Verification items for the finished model (mm, model axes). Face numbers are marked on the shaded views. A direction names the side the tool comes from. Round coordinates to 2 decimals unless told otherwise and drop trailing zeros. Write each loop counter-clockwise with the first axis right and the second up, starting at its lowest first coordinate (ties: lowest second). Pieces come first, ordered by that corner, then holes.
Autodesk Inventor part; units mm, degrees
ref_plane "YZ Plane" through (0, 0, 0) normal (1, 0, 0) x (0, 1, 0)
ref_plane "XZ Plane" through (0, 0, 0) normal (0, 1, 0) x (-1, 0, 0)
ref_plane "XY Plane" through (0, 0, 0) normal (0, 0, 1) x (1, 0, 0)
sketch "Sketch1" plane through (0, 0, 0) normal (0, 1, 0) x (-1, 0, 0)
  line L0 (55.925, 58.5) -> (-55.925, 58.5)
  line L1 (-55.925, 58.5) -> (-55.925, -58.5)
  line L2 (-55.925, -58.5) -> (55.925, -58.5)
  line L3 (55.925, -58.5) -> (55.925, 58.5)
  line L4 (55.925, 58.5) -> (-55.925, -58.5) construction
  line L5 (-55.925, 58.5) -> (55.925, -58.5) construction
  point P0 (0, 0)
  dimension "d0" = 111.85
  dimension "d1" = 117
extrude "Extrusion1" add sketch "Sketch1" along normal blind 34.19
fillet "Fillet1" radius 2 4 edges at (0, 34.19, 58.5) (55.925, 34.19, 0) (0, 34.19, -58.5) (-55.925, 34.19, 0)
sketch "Sketch2" plane through (0, 0, 0) normal (0, -1, 0) x (1, 0, 0)
  circle A0 centre (45.425, 48) radius 5.375
  line L0 (55.925, 58.5) -> (55.925, -58.5)
  line L1 (-55.925, 58.5) -> (55.925, 58.5)
  circle A1 centre (-45.575, 48) radius 5.375
  circle A2 centre (45.425, -47) radius 5.375
  circle A3 centre (-45.575, -47) radius 5.375
  point P0 (0, 0)
  dimension "d5" = 10.75
  dimension "d6" = 10.5
  dimension "d7" = 10.5
  dimension "d10" = 91
  dimension "d13" = 95
extrude "Extrusion2" add sketch "Sketch2" along normal blind 1.5
sketch "Sketch4" plane through (0, 0, 0) normal (0, -1, 0) x (1, 0, 0)
  line L0 (-55.925, -58.5) -> (-55.925, 58.5)
  line L1 (-55.925, 58.5) -> (55.925, 58.5)
  point P0 (0, 0)
  point P1 (-42.625, 0)
  dimension "d32" = 13.3
  dimension "d33" = 58.5
hole "Hole2" at (-42.625, 0, 0) direction (0, 1, 0) diameter 3 depth 1 tip angle 118
pattern_linear "Rectangular Pattern1" count 2 spacing 84.5 along (1, 0, 0) of "Hole2"
sketch "Sketch5" plane through (55.925, 0, 58.5) normal (1, 0, 0) x (0, 0, -1)
  line L0 (34.3, 14.5) -> (47.9, 14.5)
  line L1 (47.9, 14.5) -> (47.9, 8.6)
  line L2 (47.9, 8.6) -> (34.3, 8.6)
  line L3 (34.3, 8.6) -> (34.3, 14.5)
  line L4 (34.3, 14.5) -> (47.9, 8.6) construction
  line L5 (47.9, 14.5) -> (34.3, 8.6) construction
  line L6 (52.76, 14.5) -> (66.36, 14.5)
  line L7 (66.36, 14.5) -> (66.36, 8.6)
  line L8 (66.36, 8.6) -> (52.76, 8.6)
  line L9 (52.76, 8.6) -> (52.76, 14.5)
  line L10 (52.76, 14.5) -> (66.36, 8.6) construction
  line L11 (66.36, 14.5) -> (52.76, 8.6) construction
  line L12 (0, 0) -> (117, 0)
  line L13 (0, 0) -> (0, 32.19)
  point P0 (58.5, 0)
  point P1 (41.1, 11.55)
  point P2 (59.56, 11.55)
  dimension "d37" = 13.6
  dimension "d38" = 5.9
  dimension "d39" = 13.6
  dimension "d40" = 5.9
  dimension "d41" = 8.6
  dimension "d42" = 34.3
  dimension "d43" = 4.86
  dimension "d44" = 8.6
extrude "Extrusion3" cut sketch "Sketch5" against normal blind 1.5
sketch "Sketch6" plane through (55.925, 0, 58.5) normal (1, 0, 0) x (0, 0, -1)
  line L0 (66.36, 14.5) -> (66.36, 8.6)
  line L1 (0, 0) -> (117, 0)
  point P0 (58.5, 0)
  point P1 (75.26, 12)
  dimension "d54" = 8.9
  dimension "d55" = 12
hole "Hole3" at (55.925, 12, -16.76) direction (-1, 0, 0) diameter 4.24 depth 10.688 tip angle 118
sketch "Sketch7" plane through (-55.925, 0, -58.5) normal (-1, 0, 0) x (0, 0, 1)
  line L0 (0, 0) -> (117, 0)
  line L1 (0, 0) -> (0, 32.19)
  point P0 (58.5, 0)
  point P1 (20, 9.25)
  dimension "d56" = 9.25
  dimension "d64" = 20
hole "Hole4" at (-55.925, 9.25, -38.5) direction (1, 0, 0) diameter 6.88 depth 10.688 tip angle 118
sketch "Sketch8" plane through (-55.925, 0, -58.5) normal (-1, 0, 0) x (0, 0, 1)
  line L0 (33.6837, 13.1926) -> (42.498, 13.1926)
  line L1 (46.62, 11.6426) -> (46.62, 8.31)
  line L2 (46.62, 8.31) -> (30.5, 8.31)
  line L3 (30.5, 8.31) -> (30.5, 11.6426)
  line L4 (30.5, 14.87) -> (46.62, 8.31) construction
  line L5 (46.62, 14.87) -> (30.5, 8.31) construction
  circle A0 centre (20, 9.25) radius 3.44
  line L6 (0, 0) -> (117, 0)
  line L7 (30.5, 11.6426) -> (33.6837, 13.1926)
  line L8 (42.498, 13.1926) -> (46.62, 11.6426)
  point P0 (58.5, 0)
  point P1 (38.56, 11.59)
  dimension "d65" = 16.12
  dimension "d66" = 6.56
  dimension "d67" = 10.5
  dimension "d68" = 8.31
  dimension "d69" = 1.55
  dimension "d70" = 1.55
  dimension "d71" = 8.8143
extrude "Extrusion4" cut sketch "Sketch8" against normal blind 1.5 contours L0 L8 L1 L2 L3 L7
sketch "Sketch10" plane through (-55.925, 0, -58.5) normal (-1, 0, 0) x (0, 0, 1)
  line L0 (51.62, 18.8) -> (67.17, 18.8)
  line L1 (67.17, 18.8) -> (67.17, 7.1)
  line L2 (67.17, 7.1) -> (51.62, 7.1)
  line L3 (51.62, 7.1) -> (51.62, 18.8)
  line L4 (51.62, 18.8) -> (67.17, 7.1) construction
  line L5 (67.17, 18.8) -> (51.62, 7.1) construction
  line L6 (46.62, 11.6426) -> (46.62, 8.31)
  line L7 (0, 0) -> (117, 0)
  point P0 (58.5, 0)
  point P1 (59.395, 12.95)
  dimension "d81" = 15.55
  dimension "d82" = 11.7
  dimension "d84" = 5
  dimension "d85" = 7.1
extrude "Extrusion5" cut sketch "Sketch10" against normal blind 1.5
sketch "Sketch11" plane through (-55.925, 0, -58.5) normal (-1, 0, 0) x (0, 0, 1)
  line L0 (71.57, 20.05) -> (85.87, 20.05)
  line L1 (85.87, 20.05) -> (85.87, 13.45)
  line L2 (85.87, 13.45) -> (71.57, 13.45)
  line L3 (71.57, 13.45) -> (71.57, 20.05)
  line L4 (71.57, 20.05) -> (85.87, 13.45) construction
  line L5 (85.87, 20.05) -> (71.57, 13.45) construction
  line L6 (0, 32.19) -> (117, 32.19)
  line L7 (67.17, 18.8) -> (67.17, 7.1)
  line L8 (71.57, 11.05) -> (85.87, 11.05)
  line L9 (85.87, 11.05) -> (85.87, 4.45)
  line L10 (85.87, 4.45) -> (71.57, 4.45)
  line L11 (71.57, 4.45) -> (71.57, 11.05)
  point P0 (58.5, 0)
  point P1 (78.72, 16.75)
  point P2 (79.72, 17.75)
  dimension "d88" = 14.3
  dimension "d89" = 6.6
  dimension "d90" = 12.14
  dimension "d91" = 4.4
  dimension "d92" = 14.3
  dimension "d93" = 6.6
  dimension "d94" = 2.4
  dimension "d95" = 4.4
extrude "Extrusion6" cut sketch "Sketch11" against normal blind 1.5
sketch "Sketch12" plane through (-55.925, 0, -58.5) normal (-1, 0, 0) x (0, 0, 1)
  line L0 (93.15, 19.5997) -> (99.7593, 19.5997) construction
  line L1 (93.15, 17.8293) -> (99.7593, 17.8293)
  line L2 (99.7593, 21.37) -> (93.15, 21.37)
  arc A0 (93.15, 21.37) -> (93.15, 17.8293) centre (93.15, 19.5997) ccw
  arc A1 (99.7593, 17.8293) -> (99.7593, 21.37) centre (99.7593, 19.5997) ccw
  line L3 (0, 32.19) -> (117, 32.19)
  line L4 (85.87, 20.05) -> (85.87, 13.45)
  point P0 (58.5, 0)
  point P1 (96.4547, 19.5997)
  dimension "d98" = 10.15
  dimension "d99" = 10.82
  dimension "d100" = 7.28
extrude "Extrusion7" cut sketch "Sketch12" against normal blind 1.5
sketch "Sketch13" plane through (55.925, 0, 58.5) normal (1, 0, 0) x (0, 0, -1)
  line L0 (89.56, 16.8) -> (98.76, 16.8)
  line L1 (98.76, 16.8) -> (98.76, 7.6)
  line L2 (98.76, 7.6) -> (89.56, 7.6)
  line L3 (89.56, 7.6) -> (89.56, 16.8)
  line L4 (89.56, 16.8) -> (98.76, 7.6) construction
  line L5 (98.76, 16.8) -> (89.56, 7.6) construction
  circle A0 centre (75.26, 12) radius 2.12
  line L6 (0, 0) -> (117, 0)
  point P0 (58.5, 0)
  point P1 (94.16, 12.2)
  dimension "d103" = 14.3
  dimension "d104" = 7.6
  dimension "d105" = 9.2
  dimension "d106" = 9.2
extrude "Extrusion8" add sketch "Sketch13" along normal blind 1.5 contours L0 L1 L2 L3
sketch "Sketch14" plane through (-55.925, 0, 58.5) normal (0, 0, 1) x (1, 0, 0)
  line L0 (66.65, 18.82) -> (90.15, 18.82)
  line L1 (90.15, 18.82) -> (90.15, 12.25)
  line L2 (90.15, 12.25) -> (66.65, 12.25)
  line L3 (66.65, 12.25) -> (66.65, 18.82)
  line L4 (66.65, 18.82) -> (90.15, 12.25) construction
  line L5 (90.15, 18.82) -> (66.65, 12.25) construction
  line L6 (0, 0) -> (111.85, 0)
  line L7 (111.85, 0) -> (111.85, 32.19)
  point P0 (55.925, 0)
  point P1 (78.4, 15.535)
  dimension "d109" = 23.5
  dimension "d110" = 6.57
  dimension "d111" = 12.25
  dimension "d112" = 21.7
extrude "Extrusion9" cut sketch "Sketch14" against normal blind 1.5
properties part number "NUC_model"
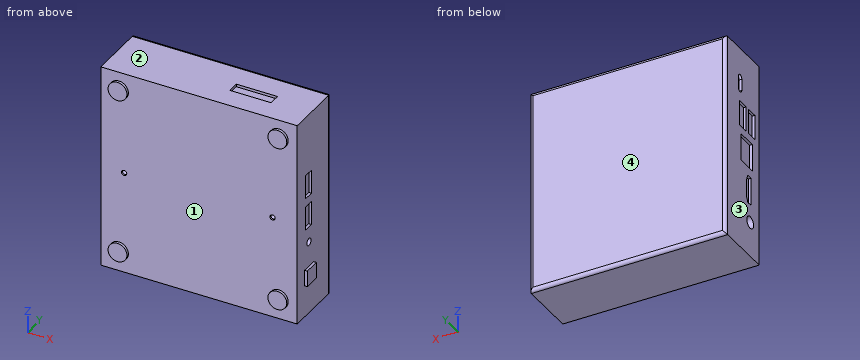
Q1. Sectioned sample at B-B (x = 28.5). Enter the section's corners in (y, z).
Recorded:
outline: (0, -58.5) - (32.19, -58.5) arc R2 ccw to (34.19, -56.5) - (34.19, 56.5) arc R2 ccw to (32.19, 58.5) - (18.82, 58.5) - (18.82, 57) - (12.25, 57) - (12.25, 58.5) - (0, 58.5) - close
Q2. Depth check by flat-ended pin: P1, Ø12, axis at x = -42, z = 9.5, coming from the -Y side; P2, Ø1.2, axis at x = -55, z = 21.5, coming from the +Y side; P3, Ø10, axis at y = 23, z = -25, coming from the +X side (3 decimals). Enter the tip coordinate at first touch or a pass-through.
Recorded:
P1: stops at y = 0
P2: stops at y = 34.13
P3: stops at x = 55.925
Q3. Sectioned sample at C-C (x = 49). Enter the section's corners in (y, z).
Recorded:
outline: (-1.5, -51.01) - (0, -51.01) - (0, -58.5) - (32.19, -58.5) arc R2 ccw to (34.19, -56.5) - (34.19, 56.5) arc R2 ccw to (32.19, 58.5) - (0, 58.5) - (0, 52.01) - (-1.5, 52.01) - (-1.5, 43.99) - (0, 43.99) - (0, -42.99) - (-1.5, -42.99) - close; hole circle Ø4.24 at (12, -16.76)
Q4. Tool access check on the marked faces 1 and 2. Record the directions out of +Z, -Z, +X, -X, +Y, -Y that give a thin tool (end or side, any length) a straight path to the whole face; none if there is none.
Recorded:
face 1: -Y
face 2: +Z, +X, -X, +Y, -Y
Q5. Material ranges on line 1 along X through (y, z) = (2.5, 46.5) (3 decimals); line 2 along Z through (x, y) = (-49, 9); line 3 along Y through (x, z) = (52, -16.76), recorded low to high.
Recorded:
line 1: x = -55.925 to 55.925
line 2: z = -58.5 to -41.93, -35.07 to 58.5
line 3: y = 0 to 9.88, 14.12 to 34.19
Q6. Sectioned sample at A-A (z = 48). Enter the section's corners in (x, y) (3 decimals).
Recorded:
outline: (-55.925, 0) - (-50.95, 0) - (-50.95, -1.5) - (-40.2, -1.5) - (-40.2, 0) - (40.05, 0) - (40.05, -1.5) - (50.8, -1.5) - (50.8, 0) - (55.925, 0) - (55.925, 32.19) arc R2 ccw to (53.925, 34.19) - (-53.925, 34.19) arc R2 ccw to (-55.925, 32.19) - close
Q7. Release check for a two-part mould opening along X. For the marked faces 3 and 4 record: released by +X, released by -X, zero draft, split by the parting line, or undercut.
Recorded:
face 3: released by -X
face 4: zero draft
Q8. Sectioned sample at D-D (z = 22). Enter the section's corners in (x, y) (3 decimals).
Recorded:
outline: (-55.925, 0) - (55.925, 0) - (55.925, 8.6) - (54.425, 8.6) - (54.425, 14.5) - (55.925, 14.5) - (55.925, 32.19) arc R2 ccw to (53.925, 34.19) - (-53.925, 34.19) arc R2 ccw to (-55.925, 32.19) - (-55.925, 20.05) - (-54.425, 20.05) - (-54.425, 13.45) - (-55.925, 13.45) - (-55.925, 11.05) - (-54.425, 11.05) - (-54.425, 4.45) - (-55.925, 4.45) - close
